Verification items for the finished model (mm, model axes). Face numbers are marked on the shaded views. Give positions to 0.01 mm unless a question says otherwise; leave off trailing zeros. Loops run counter-clockwise (first coordinate to the right, second up) from the corner with the lowest first, then second, coordinate; pieces in that order, holes last. Notation, with made-up numbers: (-4, 18) - (10, 18) arc R19 ccw to (10, 50) - close; hole circle Ø1 at (11, -37.75). An arc over 180 degrees is marked (long way). Answer in a Markdown table with one row per item.
```python
from build123d import *

# Parameters (mm, degrees)
SKETCH1_W                         = 254
SKETCH1_H                         = 114.3
BOSS_EXTRUDE1_DEPTH               = 6.35
FILLET1_R                         = 2
SKETCH6_W                         = 25
SKETCH6_H                         = 5
CUT_EXTRUDE1_DEPTH                = 140.411064841
FILLET2_R                         = 0.75
F_3_8_CLEARANCE_HOLE1_D           = 10.31748
F_3_8_CLEARANCE_HOLE1_CSINK_D     = 11.58748
F_3_8_CLEARANCE_HOLE1_CSINK_ANGLE = 90
SKETCH10_R                        = 8
CUT_EXTRUDE2_DEPTH                = 140.411064841
M3_CLEARANCE_HOLE1_D              = 5.3
M3_CLEARANCE_HOLE1_CSINK_D        = 5.35
M3_CLEARANCE_HOLE1_CSINK_ANGLE    = 90


with BuildPart() as part:
    # Sketch1 → Boss-Extrude1 (new body)
    with BuildSketch(Plane(origin=(0, 0, 0), x_dir=(1, 0, 0), z_dir=(0, 1, 0))):
        Rectangle(SKETCH1_W, SKETCH1_H)
    extrude(amount=BOSS_EXTRUDE1_DEPTH)

    # Fillet1
    fillet1_edges = [part.edges().sort_by_distance(p)[0] for p in [
        (127, 3.175, 57.15),
        (-127, 3.175, 57.15),
        (-127, 3.175, -57.15),
        (127, 3.175, -57.15),
    ]]
    fillet(fillet1_edges, radius=FILLET1_R)

    # Sketch6 → Cut-Extrude1 (cut, through all)
    with BuildSketch(Plane(origin=(0, 6.35, 0), x_dir=(1, 0, 0), z_dir=(0, 1, 0))):
        with Locations((0, 27.5)):
            Rectangle(SKETCH6_W, SKETCH6_H)
        with Locations((0, -27.5)):
            Rectangle(SKETCH6_W, SKETCH6_H)
    extrude(amount=-CUT_EXTRUDE1_DEPTH, mode=Mode.SUBTRACT)

    # Fillet2
    fillet2_edges = [part.edges().sort_by_distance(p)[0] for p in [
        (12.5, 3.175, 25),
        (12.5, 3.175, 30),
        (-12.5, 3.175, 30),
        (-12.5, 3.175, 25),
        (12.5, 3.175, -25),
        (-12.5, 3.175, -25),
        (-12.5, 3.175, -30),
        (12.5, 3.175, -30),
    ]]
    fillet(fillet2_edges, radius=FILLET2_R)

    # 3/8 Clearance Hole1 (through all)
    with Locations(Plane(origin=(0, 6.35, 0), x_dir=(1, 0, 0), z_dir=(0, 1, 0))):
        with Locations((112.7125, 42.8625), (112.7125, -42.8675), (-112.7175, 42.8625), (-112.7175, -42.8675)):
            CounterSinkHole(F_3_8_CLEARANCE_HOLE1_D / 2, F_3_8_CLEARANCE_HOLE1_CSINK_D / 2, counter_sink_angle=F_3_8_CLEARANCE_HOLE1_CSINK_ANGLE)

    # Sketch10 → Cut-Extrude2 (cut, through all)
    with BuildSketch(Plane(origin=(0, 6.35, 0), x_dir=(1, 0, 0), z_dir=(0, 1, 0))):
        with Locations(Location((-107.475, 0, 0), (0, 0, 270))):
            Circle(SKETCH10_R)
    extrude(amount=-CUT_EXTRUDE2_DEPTH, mode=Mode.SUBTRACT)

    # M3 Clearance Hole1 (through all)
    with Locations(Plane(origin=(0, 6.35, 0), x_dir=(1, 0, 0), z_dir=(0, 1, 0))):
        with Locations((-77.95, 22.1), (-77.95, -22.1)):
            CounterSinkHole(M3_CLEARANCE_HOLE1_D / 2, M3_CLEARANCE_HOLE1_CSINK_D / 2, counter_sink_angle=M3_CLEARANCE_HOLE1_CSINK_ANGLE)


solid = part.part
```
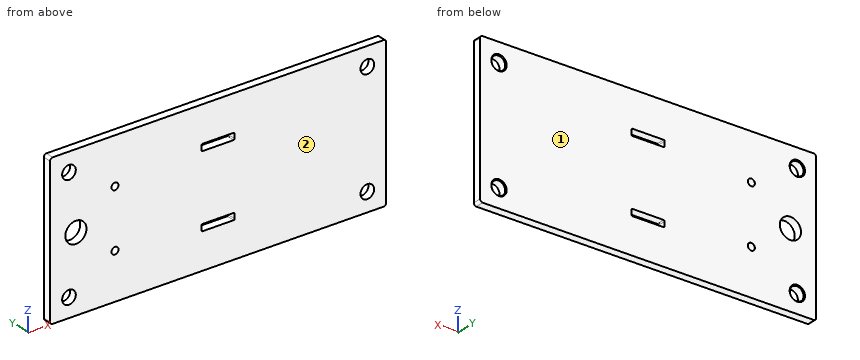
Q1. Sectioned sample at B-B (z = -22.1). Record the cut outline in (x, y) (3 decimals).
Completed:
| item | result |
|---|---|
| outline | (-127, 0) - (-80.6, 0) - (-80.6, 6.325) - (-80.625, 6.35) - (-127, 6.35) - close; (-75.3, 0) - (127, 0) - (127, 6.35) - (-75.275, 6.35) - (-75.3, 6.325) - close |
Q2. Go/stop test with a flat-tipped pin: P1, Ø7, axis at x = -77.95, z = -22.1, coming from the +Y side. Record where the tip stops, or that it passes through.
Completed:
| item | result |
|---|---|
| P1 | y = 6.35 |
Q3. Sectioned sample at C-C (y = 2.5). Give the number of separate pieces and of enclosed holes in the cut face, and give its area (3 significant figures).
Completed:
| item | result |
|---|---|
| separate pieces | 1 |
| enclosed holes | 9 |
| area | 28,200 mm^2 |
Q4. Sectioned sample at A-A (x = -77.95). Record the cut outline in (y, z) (3 decimals), and give its area (3 significant figures).
Completed:
| item | result |
|---|---|
| outline | (0, -57.15) - (6.35, -57.15) - (6.35, -24.775) - (6.325, -24.75) - (0, -24.75) - close; (0, -19.45) - (6.325, -19.45) - (6.35, -19.425) - (6.35, 19.425) - (6.325, 19.45) - (0, 19.45) - close; (0, 24.75) - (6.325, 24.75) - (6.35, 24.775) - (6.35, 57.15) - (0, 57.15) - close |
| area | 658 mm^2 |
Q5. Draft check along Y on the marked faces 1 and 2. Enter one of: +Y half, -Y half, draft (parallel to the pull), parting line (faces both ways), or undercut.
Completed:
| item | result |
|---|---|
| face 1 | +Y half |
| face 2 | -Y half |
Q6. Thickness scan on line 1 (Z direction, x = -77.95, y = 2); line 2 (X direction, y = 5.75, z = 42); line 3 (X direction, y = 1.25, z = 26). Record the ranges inside material, lowest first.
Completed:
| item | result |
|---|---|
| line 1 | -57.15 to -24.75, -19.45 to 19.45, 24.75 to 57.15 |
| line 2 | -127 to -117.84, -107.6 to 107.59, 117.83 to 127 |
| line 3 | -127 to -12.5, 12.5 to 127 |
